CAD build for the part. Positions are in the model's coordinates, mm. Face numbers are marked on the shaded views. A direction names the side the tool comes from. Round coordinates to 2 decimals unless told otherwise and drop trailing zeros. Loops run counter-clockwise (first coordinate to the right, second up) from the corner with the lowest first, then second, coordinate; pieces in that order, holes last. Notation, with made-up numbers: M 77.5,9 L 131.5,9 A25 ccw 131.5,47 Z; hole C 66.5,53.25 d11. An arc over 180 degrees is marked long. Use one line per item in the form item = value.
from build123d import *

# Parameters (mm, degrees)
F0_W     = 30.48
F0_H     = 38.1
F1_DEPTH = 88.9
F2_W     = 22.86
F2_H     = 25.4
F3_DEPTH = 152.4
F4_R     = 11.43
F5_DEPTH = 22.86
F6_W     = 36.83582
F6_H     = 53.741386
F7_DEPTH = 12.7
F8_DEPTH = 12.7


with BuildPart() as f1:
    # F0 (on Top) → F1 (new body)
    with BuildSketch(Plane.XY):
        Rectangle(F0_W, F0_H)
    extrude(amount=F1_DEPTH)

    # F2 (on face) → F3 (join)
    with BuildSketch(Plane.XY.offset(88.9)):
        Rectangle(F2_W, F2_H)
    extrude(amount=F3_DEPTH)

    # F4 (on face) → F5 (join)
    with BuildSketch(Plane(origin=(0, 0, 0), x_dir=(1, 0, 0), z_dir=(0, 0, -1))):
        Circle(F4_R)
    extrude(amount=F5_DEPTH)

    # F6 (on Right) → F7 (join)
    with BuildSketch(Plane.YZ):
        with Locations((0, -49.730693)):
            Rectangle(F6_W, F6_H)
    extrude(amount=F7_DEPTH)

    # F6 (on Right) → F8 (join)
    with BuildSketch(Plane.YZ):
        with Locations((0, -49.730693)):
            Rectangle(F6_W, F6_H)
    extrude(amount=-F8_DEPTH)


solid = f1.part
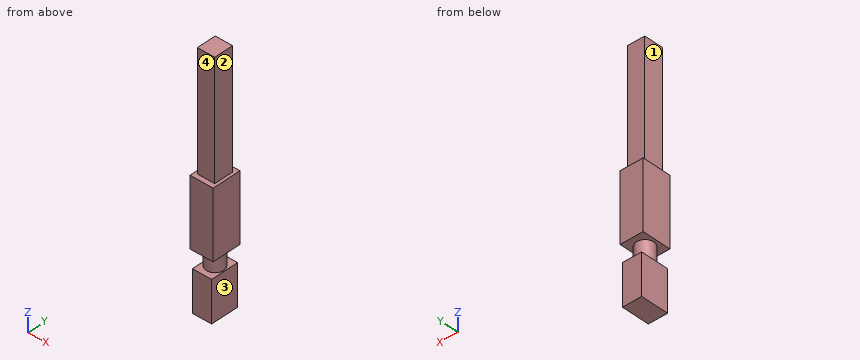
1. Probe line 1 along Z through (x, y) = (10, -7.5); line 2 along Z through (x, y) = (4, 16); line 3 along X through (y, z) = (12, 117). List the from-to ranges inside material, lowest first. Write a range as from..to.
Completed:
line_1 = -76.6..-22.86, 0..241.3
line_2 = -76.6..-22.86, 0..88.9
line_3 = -11.43..11.43
2. Drop flat-ended pins along their axis: P1, Ø20.5, axis at y = -2.5, z = 167, coming from the +X side; P2, Ø7, axis at x = 3, z = 153.5, coming from the -Y side; P3, Ø12.5, axis at x = -5, z = -44.5, coming from the -Y side. Give the stop position or say it passes through.
Completed:
P1 = 11.43
P2 = -12.7
P3 = -18.42
3. Cut at D-D on z = -19.5. Write the cut outline in (x, y), and give its area (3 significant figures).
Completed:
outline = C 0,0 d22.86
area = 410 mm2
4. Cut at A-A on y = 0. Write the cut outline in (x, z), and give its area (3 significant figures).
Completed:
outline = M -15.24,0 L -11.43,0 L -11.43,-22.86 L -12.7,-22.86 L -12.7,-76.6 L 12.7,-76.6 L 12.7,-22.86 L 11.43,-22.86 L 11.43,0 L 15.24,0 L 15.24,88.9 L 11.43,88.9 L 11.43,241.3 L -11.43,241.3 L -11.43,88.9 L -15.24,88.9 Z
area = 8,080 mm2
5. Cut at B-B on x = 0. Write the cut outline in (y, z), and give its area (3 significant figures).
Completed:
outline = M -19.05,0 L -11.43,0 L -11.43,-22.86 L -18.42,-22.86 L -18.42,-76.6 L 18.42,-76.6 L 18.42,-22.86 L 11.43,-22.86 L 11.43,0 L 19.05,0 L 19.05,88.9 L 12.7,88.9 L 12.7,241.3 L -12.7,241.3 L -12.7,88.9 L -19.05,88.9 Z
area = 9,760 mm2
6. Tool access for the marked faces 1, 2, 3 and 4: list every direction of +Z, -Z, +X, -X, +Y, -Y with a clear straight run to the whole face (end or side of a thin tool).
Completed:
face_1 = +Z, -X, +Y, -Y
face_2 = +Z, +X, +Y, -Y
face_3 = -Z, +X, +Y, -Y
face_4 = +Z, +X, -X, -Y
7. Cut at C-C on z = 174. Write the cut outline in (x, y).
Completed:
outline = M -11.43,-12.7 L 11.43,-12.7 L 11.43,12.7 L -11.43,12.7 Z
